Geometry: see drawing. Coordinates: mm, zero at the bounding-box minimum. A direction names the side the tool comes from. Give positions to 0.01 mm unless a question says otherwise; leave off trailing zeros. Loops run counter-clockwise (first coordinate to the right, second up) from the corner with the lowest first, then second, coordinate; pieces in that order, holes last. Notation, with made-up numbers: (77.5, 68) -> (130.5, 68) arc R7 ccw to (130.5, 81) -> close; hole circle Ø6 at (-28.75, -11). An arc over 180 degrees is marked (long way). Return JSON: item names as keys, results as strings. Group by question number.
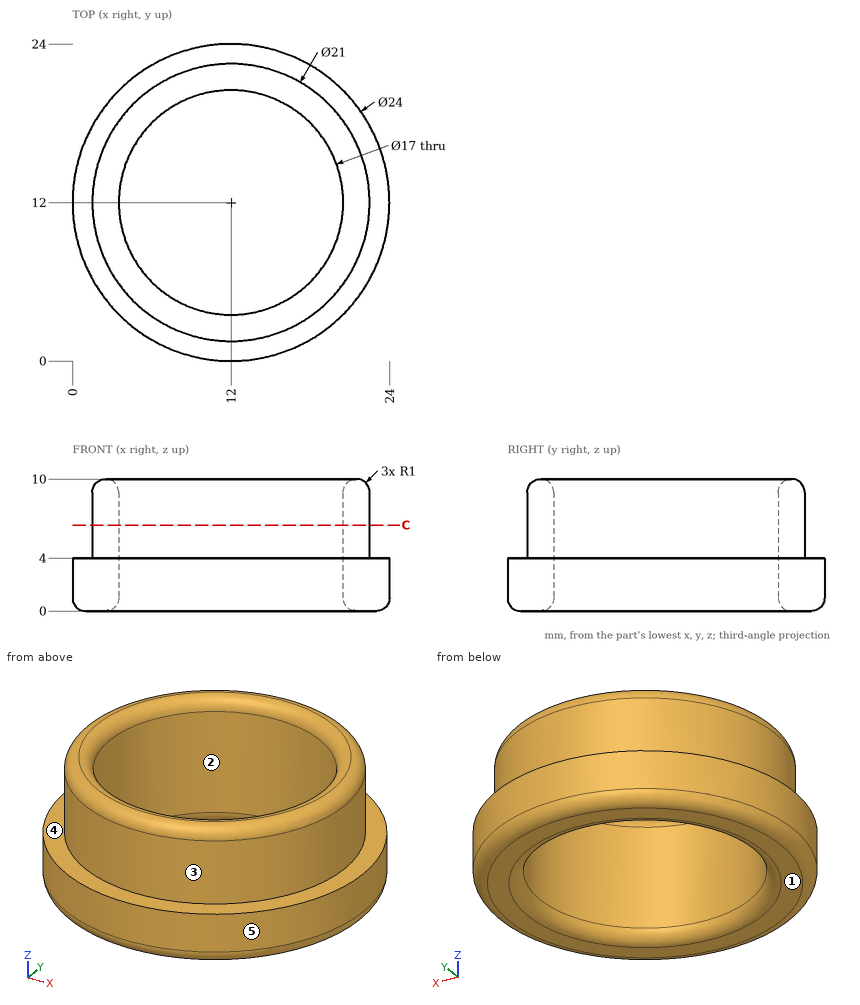
1) Cut plane C-C on z = 6.5. Return loops of the section in (x, y).
2) Reachability of the marked faces 4 and 5 from +Z, -Z, +X, -X, +Y, -Y: full face, straight path, thin tool, end or side. Return the list, or none.
3) Contact query for flat-ended pins moving along their axis: P1, Ø6, axis at x = 10, z = 8.5, coming from the +Y side; P2, Ø3, axis at x = 18.5, z = 3.5, coming from the +Y side; P3, Ø3, axis at x = 9.5, z = 6.5, coming from the -Y side. Output: stop coordinate, or through.
4) Material intervals for line 1 (Y direction, x = 12, z = 3.75); line 2 (Y direction, x = 12, z = 4.5); line 3 (X direction, y = 12.5, z = 8.5), sorted ascending.
5) Mould query, pull axis X, two halves, no side actions, for the marked faces 1, 2 and 3. Classes: released by +X, released by -X, zero draft, split by the parting line, or undercut.
Calculated:
{
 "1": {"outline": "circle Ø21 at (12, 12); hole circle Ø17 at (12, 12)"},
 "2": {"face 4": "+Z", "face 5": "+Z, -Z"},
 "3": {"P1": "y = 22.5", "P2": "y = 22.91", "P3": "y = 1.55"},
 "4": {"line 1": "0 to 3.5, 20.5 to 24", "line 2": "1.5 to 3.5, 20.5 to 22.5", "line 3": "1.51 to 3.51, 20.49 to 22.49"},
 "5": {"face 1": "zero draft", "face 2": "undercut", "face 3": "split by the parting line"}
}
